```python
from build123d import *

# Parameters (mm, degrees)
SKETCH1_W             = 158
SKETCH1_H             = 92
BOSS_EXTRUDE1_DEPTH   = 8
SKETCH2_W             = 158
SKETCH2_H             = 92
SKETCH2_W_2           = 148
SKETCH2_H_2           = 82
BOSS_EXTRUDE2_DEPTH   = 15
SKETCH3_R             = 33
CUT_EXTRUDE1_DEPTH    = 95.265582266
FILLET1_R             = 5
FILLET2_R             = 5
SPLIT1_START          = -29
SPLIT1_OUTLINE_W      = 15
SPLIT1_OUTLINE_H      = 5
SPLIT1_DEPTH          = 83
M4X0_7_TAPPED_HOLE1_D = 3.3


# Read off the part's stored shape, not the designer's step: Split1
with BuildPart() as part:
    # Sketch1 → Boss-Extrude1 (new body)
    with BuildSketch(Plane(origin=(0, 0, 0), x_dir=(1, 0, 0), z_dir=(0, 1, 0))):
        Rectangle(SKETCH1_W, SKETCH1_H)
    extrude(amount=BOSS_EXTRUDE1_DEPTH)

    # Sketch2 → Boss-Extrude2 (add)
    with BuildSketch(Plane(origin=(0, 8, 0), x_dir=(1, 0, 0), z_dir=(0, 1, 0))):
        Rectangle(SKETCH2_W, SKETCH2_H)
        Rectangle(SKETCH2_W_2, SKETCH2_H_2, mode=Mode.SUBTRACT)
    extrude(amount=BOSS_EXTRUDE2_DEPTH)

    # Sketch3 → Cut-Extrude1 (cut, through all)
    with BuildSketch(Plane.XZ):
        with Locations(Location((0, 0, 0), (0, 0, 270))):
            Circle(SKETCH3_R)
    extrude(amount=-CUT_EXTRUDE1_DEPTH, mode=Mode.SUBTRACT)

    # Fillet1
    fillet1_edges = [part.edges().sort_by_distance(p)[0] for p in [
        (-79, 11.5, 46),
    ]]
    fillet(fillet1_edges, radius=FILLET1_R)

    # Fillet2
    fillet2_edges = [part.edges().sort_by_distance(p)[0] for p in [
        (79, 11.5, 46),
        (-79, 11.5, -46),
        (79, 11.5, -46),
    ]]
    fillet(fillet2_edges, radius=FILLET2_R)

    # Split1 outline → Split1 (cut)
    with BuildSketch(Plane.YZ.offset(SPLIT1_START)):
        with Locations((15.5, -43.5)):
            Rectangle(SPLIT1_OUTLINE_W, SPLIT1_OUTLINE_H)
    extrude(amount=SPLIT1_DEPTH, mode=Mode.SUBTRACT)

    # M4x0.7 Tapped Hole1 (through all)
    with Locations(Plane.XY.offset(46)):
        with Locations((0, 4)):
            Hole(M4X0_7_TAPPED_HOLE1_D / 2)


solid = part.part
```
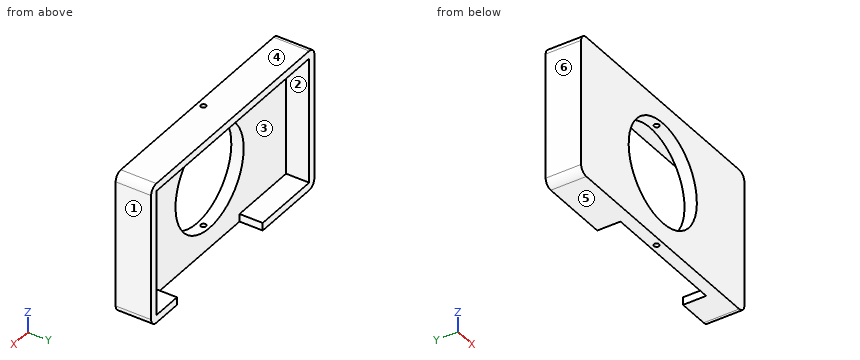
Part model, mm, in its own coordinate system. Face numbers are marked on the shaded views. A direction names the side the tool comes from. Coordinates: 2 decimals unless noted, no trailing zeros. Loops run counter-clockwise (first coordinate to the right, second up) from the corner with the lowest first, then second, coordinate; pieces in that order, holes last. Notation, with made-up numbers: (-27, 74.5) - (-23, 74.5) arc R11 cw to (-23, 80.5) - close; hole circle Ø1 at (-8, 69.25). An arc over 180 degrees is marked (long way). Write item = value, one per line. Start each with the question number.
Item 1: Cut at A-A, the plane y = 4. Give the cut face in (x, z).
Item 2: Cut at B-B, the plane x = 0. Give the cut face in (y, z), and give its area (3 significant figures).
Item 3: Mould opens along Z. For the marked faces 3, 4, 5 and 6 say: released by +Z, released by -Z, zero draft, split by the parting line, or undercut.
Item 4: Cut at C-C, the plane z = 0. Give the cut face in (x, y).
Item 5: Wall check: L1, parallel to X at y = 4, z = 35.5; L2, parallel to X at y = 16.25, z = -7; L3, parallel to Y at x = 0, z = -35.75. Give the ranges that are in metal, low to high. Write a range as from..to.
Item 6: Cut at D-D, the plane x = 23.5. Give the cut face in (y, z).
Item 7: Flat gauge pins, fed straight in: pin 1 Ø2 at (x, z) = (-29.5, -16) entering from +Y; pin 2 Ø4 at (y, z) = (17.5, -44.5) entering from +X. Where does each tip first touch, or does it go through?
Item 8: 3-axis set-ups, long thin cutter, end or side, ignore diameter. For the marked faces 1 and 2: which of +Z, -Z, +X, -X, +Y, -Y reach the whole face in a straight line?
The answers:
q1.outline = (-79, -41) arc R5 ccw to (-74, -46) - (-1.65, -46) - (-1.65, -32.96) arc R33 cw to (-1.65, 32.96) - (-1.65, 46) - (-74, 46) arc R5 ccw to (-79, 41) - close; (1.65, -46) - (74, -46) arc R5 ccw to (79, -41) - (79, 41) arc R5 ccw to (74, 46) - (1.65, 46) - (1.65, 32.96) arc R33 cw to (1.65, -32.96) - close
q2.outline = (0, -46) - (2.35, -46) - (2.35, -33) - (0, -33) - close; (0, 33) - (2.35, 33) - (2.35, 46) - (0, 46) - close; (5.65, -46) - (8, -46) - (8, -33) - (5.65, -33) - close; (5.65, 33) - (8, 33) - (8, 41) - (23, 41) - (23, 46) - (5.65, 46) - close
q2.area = 197 mm2
q3.face_3 = undercut
q3.face_4 = released by +Z
q3.face_5 = released by -Z
q3.face_6 = zero draft
q4.outline = (-79, 0) - (-33, 0) - (-33, 8) - (-74, 8) - (-74, 23) - (-79, 23) - close; (33, 0) - (79, 0) - (79, 23) - (74, 23) - (74, 8) - (33, 8) - close
q5.L1 = -79..-1.65, 1.65..79
q5.L2 = -79..-74, 74..79
q5.L3 = 0..2.35, 5.65..8
q6.outline = (0, -46) - (8, -46) - (8, -23.17) - (0, -23.17) - close; (0, 23.17) - (8, 23.17) - (8, 41) - (23, 41) - (23, 46) - (0, 46) - close
q7.pin_1 = 8
q7.pin_2 = 78.77
q8.face_1 = +Z, -Z, +X, +Y, -Y
q8.face_2 = +Y
